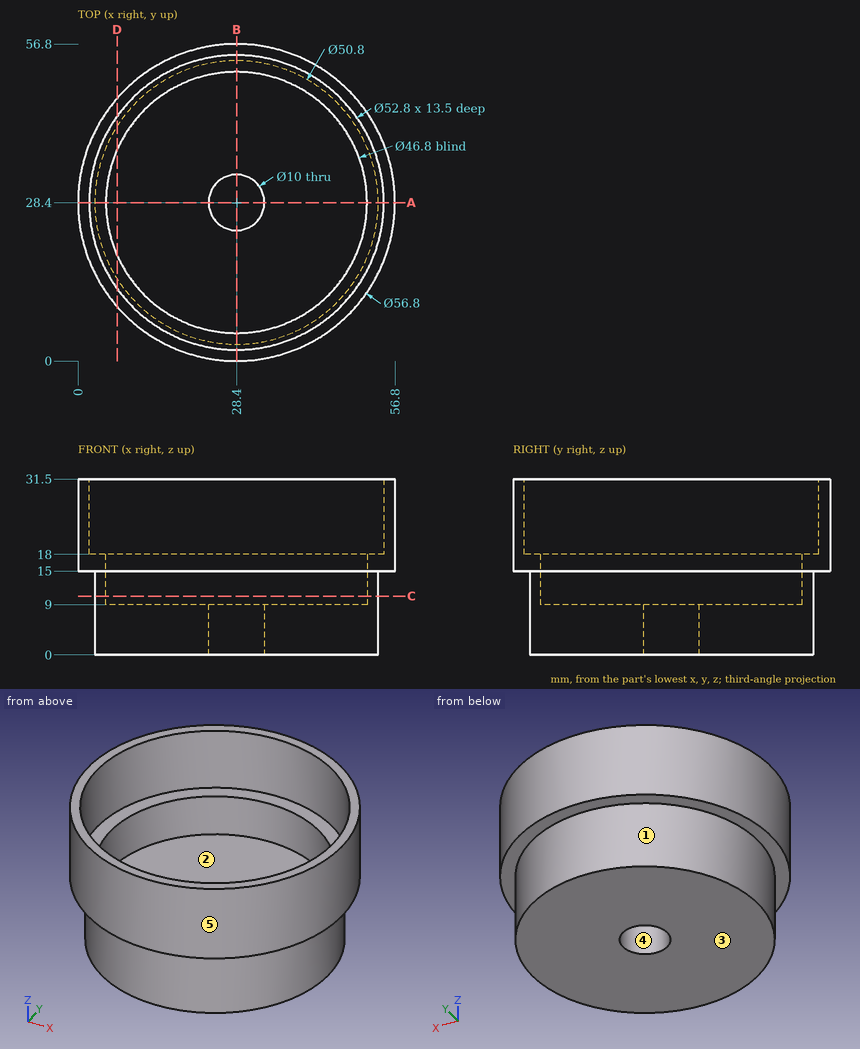
Could you check a few things on this drawing? It's one solid part, dimensions in mm from its lowest x, y, z. A direction names the side the tool comes from. Coordinates: 2 decimals unless noted, no trailing zeros. Order: outer loops, then holes, each group sorted by start corner. A loop starts at its lowest first (then second) coordinate and runs counter-clockwise, first axis right, second up. Notation, with made-up numbers: M -6.5,50.25 L 14.5,50.25 A10 ccw 14.5,65.25 Z; hole C 23.5,-29.75 d1. An arc over 180 degrees is marked long. Use a Markdown table: item, result. Add a question column.
Q1. I want a section at C-C on z = 10.5. List the corners of the cut face in (x, y) for me.
Q2. I'm going to push flat-ended pins straight in: pin 1 (23.5 mm diameter, centred on x = 36, y = 30, fed in from +Z); pin 2 (10 mm diameter, centred on x = 15.5, y = 43.5, fed in from +Z); pin 3 (6 mm diameter, centred on x = 28.4, y = 28.4, fed in from -Z); pin 4 (1.5 mm diameter, centred on x = 28, z = 15, fed in from -Y). Where does each tip first touch, or does it pass through?
Q3. Which directions (+Z, -Z, +X, -X, +Y, -Y) give clear straight access to the entire face, cutting with the end or side of a thin tool? Please do the marked faces 1 and 2.
Q4. I want a section at D-D on x = 7. List the corners of the cut face in (y, z) for me, then the cut area to 3 significant figures.
Q5. We'd pull the mould along Y, two halves only. Please class the marked faces 3, 4 and 5: pulls with the +Y half, pulls with the -Y half, needs draft (parallel to the pull), parting line crosses it, or undercut.
Q6. I want a section at A-A on y = 28.4. List the corners of the cut face in (x, z) for me.
Q7. If I drill on L1, parallel to Y at x = 28.4, z = 23; L2, parallel to X at y = 28, z = 14; L3, parallel to Y at x = 28.4, z = 6.5, over which ranges is the centre line in solid material (lowest first)?
Checked values:
| question | item | result |
|---|---|---|
| 1 | outline | C 28.4,28.4 d50.8; hole C 28.4,28.4 d46.8 |
| 2 | pin 1 | z = 9 |
| 2 | pin 2 | z = 18 |
| 2 | pin 3 | through |
| 2 | pin 4 | y = 0 |
| 3 | face 1 | -Z |
| 3 | face 2 | +Z |
| 4 | outline | M 9.73,15 L 14.72,15 L 14.72,0 L 42.08,0 L 42.08,15 L 47.07,15 L 47.07,31.5 L 43.86,31.5 L 43.86,18 L 37.87,18 L 37.87,9 L 18.93,9 L 18.93,18 L 12.94,18 L 12.94,31.5 L 9.73,31.5 Z |
| 4 | area | 439 mm² |
| 5 | face 3 | needs draft |
| 5 | face 4 | undercut |
| 5 | face 5 | parting line crosses it |
| 6 | outline | M 0,15 L 3,15 L 3,0 L 23.4,0 L 23.4,9 L 5,9 L 5,18 L 2,18 L 2,31.5 L 0,31.5 Z; M 33.4,0 L 53.8,0 L 53.8,15 L 56.8,15 L 56.8,31.5 L 54.8,31.5 L 54.8,18 L 51.8,18 L 51.8,9 L 33.4,9 Z |
| 7 | L1 | 0 to 2, 54.8 to 56.8 |
| 7 | L2 | 3 to 5, 51.8 to 53.8 |
| 7 | L3 | 3 to 23.4, 33.4 to 53.8 |
